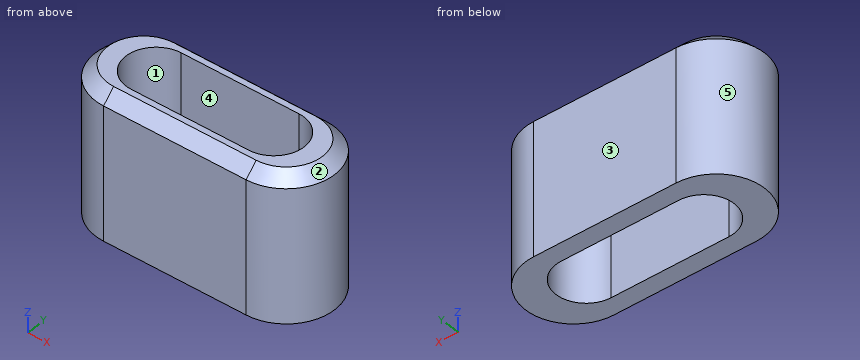
from build123d import *

# Parameters (mm, degrees)
F1_DEPTH = 60
F2_SIZE2 = 5
F2_SIZE  = 5


with BuildPart() as f1:
    # F0 (on Top) → F1 (new body)
    with BuildSketch(Plane.XY):
        with BuildLine():
            Line((30, 20), (0, 20))
            Line((0, 20), (-30, 20))
            ThreePointArc((-30, 20), (-50, 0), (-30, -20))
            Line((-30, -20), (0, -20))
            Line((0, -20), (30, -20))
            ThreePointArc((30, -20), (50, 0), (30, 20))
        make_face()
        with BuildLine():
            Line((-30, 15), (0, 15))
            Line((0, 15), (30, 15))
            ThreePointArc((30, 15), (45, 0), (30, -15))
            Line((30, -15), (0, -15))
            Line((0, -15), (-30, -15))
            ThreePointArc((-30, -15), (-45, 0), (-30, 15))
        make_face(mode=Mode.SUBTRACT)
        with BuildLine():
            Line((30, 15), (0, 15))
            Line((0, 15), (-30, 15))
            ThreePointArc((-30, 15), (-45, 0), (-30, -15))
            Line((-30, -15), (0, -15))
            Line((0, -15), (30, -15))
            ThreePointArc((30, -15), (45, 0), (30, 15))
        make_face()
        with BuildLine():
            Line((24.7928556055, -12.5), (0, -12.5))
            Line((0, -12.5), (-24.7928556055, -12.5))
            ThreePointArc((-24.7928556055, -12.5), (-37.2928556055, 0), (-24.7928556055, 12.5))
            Line((-24.7928556055, 12.5), (0, 12.5))
            Line((0, 12.5), (24.7928556055, 12.5))
            ThreePointArc((24.7928556055, 12.5), (37.2928556055, 0), (24.7928556055, -12.5))
        make_face(mode=Mode.SUBTRACT)
    extrude(amount=F1_DEPTH)

    # F2
    f2_edges = [f1.edges().sort_by_distance(p)[0] for p in [
        (-50, 0, 60),
    ]]
    chamfer(f2_edges, length=F2_SIZE, length2=F2_SIZE2)


solid = f1.part
For this review, take the finished solid that the model builds, in its own axes (mm). Face numbers are marked on the shaded views. A direction names the side the tool comes from. Round coordinates to 2 decimals unless told otherwise and drop trailing zeros. Loops run counter-clockwise (first coordinate to the right, second up) from the corner with the lowest first, then second, coordinate; pieces in that order, holes last. Notation, with made-up numbers: (-30.5, -8) - (17.5, -8) arc R22 ccw to (17.5, 15) - close; hole circle Ø1 at (27.25, -8). An arc over 180 degrees is marked (long way). Put each result on its own line as item: value. Start each with the question number.
1. For the marked faces 4 and 5, list the 3-axis set-ups (+Z, -Z, +X, -X, +Y, -Y) from which the entire face can be reached by the end or side of a thin tool; tool diameter is ignored.
2. For probe 1 along Y at (x, z) = (3.5, 53); probe 2 along X at (y, z) = (-0.5, 49.5); probe 3 along Y at (x, z) = (-30, 37), list the stretches that pass through material, from the lowest coordinate up. Write a range as [from, to].
3. Consider section B-B on x = 10. State the section outline as (y, z) points.
4. Consider section A-A on y = 0. State the section outline as (x, z) points, plus the area to 3 significant figures.
5. Consider section C-C on z = 31. State the section outline as (x, y) points.
6. Insertion check: P1, Ø6, axis at x = -33, z = 34, coming from the -Y side; P2, Ø2, axis at y = 8.5, z = 26, coming from the +X side; P3, Ø1.5, axis at y = 0.5, z = 48, coming from the -X side. Each pin has a flat end and moves straight along its axis. Give the tip position at first contact, or say it passes through.
7. Mouldability with a two-part tool opening along Y and no side actions: class the marked faces 1, 2 and 3 as +Y half, -Y half, draft (parallel to the pull), parting line (faces both ways), or undercut.
Result sheet:
1. face 4: +Z, -Z
1. face 5: +Z, -Z, -X
2. probe 1: [-20, -12.5], [12.5, 20]
2. probe 2: [-49.99, -37.28], [37.28, 49.99]
2. probe 3: [-20, -11.36], [11.36, 20]
3. outline: (-20, 0) - (-12.5, 0) - (-12.5, 60) - (-15, 60) - (-20, 55) - close; (12.5, 0) - (20, 0) - (20, 55) - (15, 60) - (12.5, 60) - close
4. outline: (-50, 0) - (-37.29, 0) - (-37.29, 60) - (-45, 60) - (-50, 55) - close; (37.29, 0) - (50, 0) - (50, 55) - (45, 60) - (37.29, 60) - close
4. area: 1,500 mm^2
5. outline: (-30, -20) - (30, -20) arc R20 ccw to (30, 20) - (-30, 20) arc R20 ccw to start; hole (-24.79, -12.5) - (24.79, -12.5) arc R12.5 ccw to (24.79, 12.5) - (-24.79, 12.5) arc R12.5 ccw to start
6. P1: y = -20
6. P2: x = 48.54
6. P3: x = -50
7. face 1: undercut
7. face 2: parting line
7. face 3: +Y half
